from build123d import *

# Parameters (mm, degrees)
RESSALTO_EXTRUS_O1_DEPTH = 4
RESSALTO_EXTRUS_O5_DEPTH = 4
ESBO_O15_W               = 16
ESBO_O15_H               = 4.2
ESBO_O15_H_2             = 3
CORTE_EXTRUS_O2_DEPTH    = 137.905868833
CORTE_EXTRUS_O3_DEPTH    = 141.792239382
FILETE1_R                = 5
CORTE_EXTRUS_O4_DEPTH    = 141.602820342


with BuildPart() as part:
    # Esboço1 → Ressalto-extrusão1 (new body)
    with BuildSketch(Plane.XY):
        Polygon((0, 0), (0, 76), (118.45022022, 62.267517703), (115, -13.332482297), align=None)
    extrude(amount=RESSALTO_EXTRUS_O1_DEPTH)

    # Esboço13 → Ressalto-extrusão5 (add)
    with BuildSketch(Plane.XY.offset(4)):
        Polygon((0, 0), (-39.756896509, 4.609201034), (0, 76), align=None)
    extrude(amount=-RESSALTO_EXTRUS_O5_DEPTH)

    # Esboço15 → Corte-extrusão2 (cut, through all)
    with BuildSketch(Plane(origin=(10.533319004, -0.48071786, 35.325049871), x_dir=(0.045590380198121984, 0.9989602180434368, 0), z_dir=(0.28572546626048706, -0.013039891282772654, 0.9582227920298917))):
        with Locations((57.047089405, 0.914508914)):
            Rectangle(ESBO_O15_W, ESBO_O15_H)
        with Locations((26.001686631, 0.719596914)):
            Rectangle(ESBO_O15_W, ESBO_O15_H)
        with Locations((48.602963636, -108.019389568)):
            Rectangle(ESBO_O15_W, ESBO_O15_H_2)
        with Locations((17.602963636, -108.019389568)):
            Rectangle(ESBO_O15_W, ESBO_O15_H_2)
    extrude(amount=-CORTE_EXTRUS_O2_DEPTH, mode=Mode.SUBTRACT)

    # Esboço16 → Corte-extrusão3 (cut, through all)
    with BuildSketch(Plane.XY.offset(4)):
        Polygon((116.384955754, 51.350322393), (121.395369813, 51.350322393), (120.655509671, 35.138769736), (115.655509671, 35.366958904), align=None)
        Polygon((114.971653968, 20.382555633), (118.971653968, 20.200004299), (118.242207885, 4.21664081), (114.242207885, 4.399192144), align=None)
    extrude(amount=-CORTE_EXTRUS_O3_DEPTH, mode=Mode.SUBTRACT)

    # Filete1
    filete1_edges = [part.edges().sort_by_distance(p)[0] for p in [
        (-39.756896509, 4.609201034, 2),
        (0, 76, 2),
    ]]
    fillet(filete1_edges, radius=FILETE1_R)

    # Esboço19 → Corte-extrusão4 (cut, through all)
    with BuildSketch(Plane.XY.offset(4)):
        Polygon((5.394142853, 64.868617599), (0.394142853, 65.096806767), (-0.33530323, 49.113443279), (4.66469677, 48.885254111), align=None)
        Polygon((4.181969533, 33.84622174), (3.45252345, 17.862858252), (-1.54747655, 18.091047419), (-0.818030467, 34.074410908), align=None)
    extrude(amount=-CORTE_EXTRUS_O4_DEPTH, mode=Mode.SUBTRACT)


solid = part.part
Can you work these out from the model? Positions are in its coordinate system, mm. A direction names the side the tool comes from. Coordinates: 2 decimals unless noted, no trailing zeros. Write each loop counter-clockwise with the first axis right and the second up, starting at its lowest first coordinate (ties: lowest second). Pieces come first, ordered by that corner, then holes. Notation, with made-up numbers: (51.5, 12.5) -> (93.5, 12.5) arc R33 ccw to (93.5, 41.5) -> close; hole circle Ø8 at (31.25, 85). An arc over 180 degrees is marked (long way). Write each question's results on one line, items separated by ' | '. Start each with the question number.
Q1. Imagine slicing it at C-C (x = -8.5). Write out the boundary of the cut face in (y, z).
Q2. On a 3-axis mill with a long thin cutter (end or side, diameter ignored), from which of +Z, -Z, +X, -X, +Y, -Y can I reach the whole of each face in a straight line? I mean faces 1 (the face through (-19.1, 41.7, 2)), 2 (the face through (3.822, 25.966, 2.028)), 3 (the face through (115.3, 51.4, 1.9)). Say none if no direction works.
Q3. I'm going to push flat-ended pins straight in: pin 1 (1.5 mm diameter, centred on y = 16, z = 2.5, fed in from -X); pin 2 (1 mm diameter, centred on y = 49.5, z = 2, fed in from +X); pin 3 (1.5 mm diameter, centred on x = 20, z = 1.5, fed in from -Y). Where does each tip first touch, or does it pass through?
Q4. Imagine slicing it at D-D (y = 68). Write out the boundary of the cut face in (x, z), then the cut area to 3 significant figures.
Q5. Imagine slicing it at B-B (y = 59). Write out the boundary of the cut face in (x, z), then the cut area to 3 significant figures.
Q6. Imagine slicing it at A-A (z = 0.75). Write out the boundary of the cut face in (x, y).
Q7. We'd pull the mould along X, two halves only. Please class faces 4 (the face through (5.024, 56.765, 2.028)), 5 (the face through (-36.166, 6.373, 1.972)), 6 (the face through (116.882, 27.908, 1.972)), 7 (the face through (42, 32, 0)): +X half, -X half, draft (parallel to the pull), parting line (faces both ways), or undercut.
Q8. If I drill on probe 1 along X at (y, z) = (29.5, 0.2); probe 2 along X at (y, z) = (52, 1.75); probe 3 along Y at (x, z) = (2.5, 0.25), over which ranges is the centre line in solid material (lowest first)?
Taken from the geometry:
1) outline: (0.99, 0) -> (60.74, 0) -> (60.74, 4) -> (0.99, 4) -> close
2) face 1: +Z, -Z, -X, +Y | face 2: +Z, -Z | face 3: -Z
3) pin 1: stops at x = -33.83 | pin 2: stops at x = 114.29 | pin 3: stops at y = -2.41
4) outline: (-4.46, 0) -> (69, 0) -> (69, 4) -> (-4.46, 4) -> close | area: 294 mm^2
5) outline: (-9.47, 0) -> (-0.46, 0) -> (0.12, 1.92) -> (0.12, 4) -> (-9.47, 4) -> close; (5.13, 0) -> (118.3, 0) -> (118.3, 4) -> (5.13, 4) -> close | area: 490 mm^2
6) outline: (-36.12, 11.15) arc R5 ccw to (-32.32, 3.75) -> (115, -13.33) -> (115.81, 4.33) -> (111.71, 4.51) -> (112.44, 20.5) -> (116.54, 20.31) -> (117.22, 35.3) -> (113.12, 35.48) -> (113.85, 51.47) -> (116.38, 51.35) -> (117.95, 51.35) -> (118.45, 62.27) -> (3.32, 75.62) arc R5 ccw to (-1.63, 73.08) -> close; hole (-1.9, 18.11) -> (3.45, 17.86) -> (4.18, 33.85) -> (-1.17, 34.09) -> close; hole (-0.68, 49.13) -> (4.66, 48.89) -> (5.39, 64.87) -> (0.05, 65.11) -> close
7) face 4: undercut | face 5: -X half | face 6: +X half | face 7: draft
8) probe 1: x = -25.9 to -1.54, 3.98 to 116.95 | probe 2: x = -13.37 to -0.25, 4.81 to 117.98 | probe 3: y = -0.29 to 17.91, 33.92 to 48.98, 65 to 75.64
